```python
from build123d import *

# Parameters (mm, degrees)
SKIZZE1_W                       = 60
SKIZZE1_H                       = 60
AUFSATZ_LINEAR_AUSTRAGEN1_DEPTH = 3
SKIZZE3_R                       = 1.5
SKIZZE3_R_2                     = 9.5
SCHNITT_LINEAR_AUSTRAGEN2_DEPTH = 43.532340636


with BuildPart() as part:
    # Skizze1 → Aufsatz-Linear austragen1 (new body)
    with BuildSketch(Plane(origin=(0, 0, 0), x_dir=(0, 0, -1), z_dir=(1, 0, 0))):
        Rectangle(SKIZZE1_W, SKIZZE1_H)
    extrude(amount=AUFSATZ_LINEAR_AUSTRAGEN1_DEPTH)

    # Skizze3 → Schnitt-Linear austragen2 (cut, through all)
    with BuildSketch(Plane(origin=(3, 0, 0), x_dir=(0, 0, -1), z_dir=(1, 0, 0))):
        with Locations((-15, 25)):
            Circle(SKIZZE3_R)
        with Locations((15, 25)):
            Circle(SKIZZE3_R)
        Circle(SKIZZE3_R_2)
    extrude(amount=-SCHNITT_LINEAR_AUSTRAGEN2_DEPTH, mode=Mode.SUBTRACT)


solid = part.part
```
Source: CAD feature listing. Evaluate the final solid. Frame: model axes, mm. Round coordinates to 2 decimals unless told otherwise and drop trailing zeros. Loops run counter-clockwise (first coordinate to the right, second up) from the corner with the lowest first, then second, coordinate; pieces in that order, holes last.
(1) Material intervals for probe 1 along Y at (x, z) = (2.4, 0); probe 2 along Y at (x, z) = (1.3, -15); probe 3 along Z at (x, y) = (0.1, 26), sorted ascending.
From the geometry:
probe 1: y = -30 to -9.5, 9.5 to 30
probe 2: y = -30 to 23.5, 26.5 to 30
probe 3: z = -30 to -16.12, -13.88 to 13.88, 16.12 to 30
(2) Section query B-B (z = 0). Output: boundary loops of the cut face in (x, y).
From the geometry:
outline: (0, -30) - (3, -30) - (3, -9.5) - (0, -9.5) - close; (0, 9.5) - (3, 9.5) - (3, 30) - (0, 30) - close
(3) Section query C-C (x = 0.8). Output: boundary loops of the cut face in (y, z), and give its area (3 significant figures).
From the geometry:
outline: (-30, -30) - (30, -30) - (30, 30) - (-30, 30) - close; hole circle Ø19 at (0, 0); hole circle Ø3 at (25, -15); hole circle Ø3 at (25, 15)
area: 3,300 mm2
(4) Section query D-D (z = -8). Output: boundary loops of the cut face in (x, y), and give its area (3 significant figures).
From the geometry:
outline: (0, -30) - (3, -30) - (3, -5.12) - (0, -5.12) - close; (0, 5.12) - (3, 5.12) - (3, 30) - (0, 30) - close
area: 149 mm2
(5) Contact query for a flat-ended pin moving along its axis: pin 1 Ø1.8 at (y, z) = (25, -15) entering from -X. Output: stop coordinate, or through.
From the geometry:
pin 1: passes through
(6) Pull-direction query (Y, two-part tool) for faces 1 (the cylindrical face through (1.52, 26.01, 16.11)), 2 (the cylindrical face through (1.52, 26.01, -13.89)), 3 (the flat face through (1, -30, 0)), 4 (the flat face through (1, 0, 30)); classes: +Y half, -Y half, draft (parallel to the pull), parting line (faces both ways), or undercut.
From the geometry:
face 1: undercut
face 2: undercut
face 3: -Y half
face 4: draft
(7) Section query A-A (y = 25). Output: boundary loops of the cut face in (x, z), and give its area (3 significant figures).
From the geometry:
outline: (0, -30) - (3, -30) - (3, -16.5) - (0, -16.5) - close; (0, -13.5) - (3, -13.5) - (3, 13.5) - (0, 13.5) - close; (0, 16.5) - (3, 16.5) - (3, 30) - (0, 30) - close
area: 162 mm2
